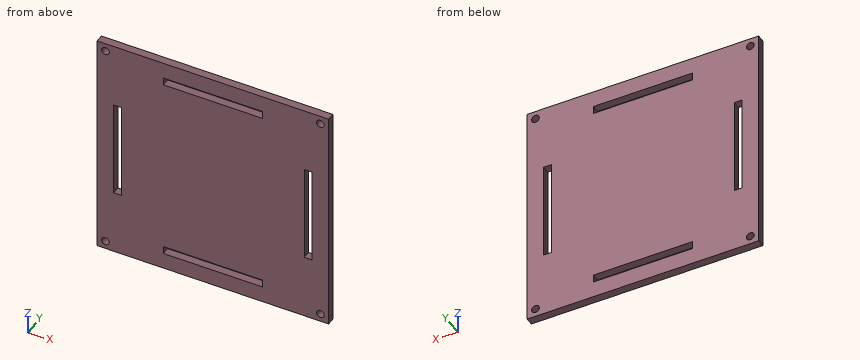
```python
from build123d import *

# Parameters (mm, degrees)
SKETCH_2_W          = 88.9
SKETCH_2_H          = 3
EXTRUDE_1_DEPTH     = 88.9
SKETCH_4_R          = 1.5
CUT_EXTRUDE_1_DEPTH = 3
SKETCH_10_W         = 3
SKETCH_10_H         = 38.1
SKETCH_10_W_2       = 38.1
SKETCH_10_H_2       = 3
CUT_EXTRUDE_6_DEPTH = 3


with BuildPart() as part:
    # 스케치2 → 보스-돌출1 (new body)
    with BuildSketch(Plane.XY):
        Rectangle(SKETCH_2_W, SKETCH_2_H)
    extrude(amount=EXTRUDE_1_DEPTH)

    # 스케치4 → 컷-돌출1 (cut)
    with BuildSketch(Plane(origin=(0, 1.5, 0), x_dir=(1, 0, 0), z_dir=(0, 1, 0))):
        with Locations(Location((-41.275, -85.725, 0), (0, 0, 270))):
            Circle(SKETCH_4_R)
        with Locations(Location((-41.275, -3.175, 0), (0, 0, 270))):
            Circle(SKETCH_4_R)
        with Locations(Location((41.275, -3.175, 0), (0, 0, 270))):
            Circle(SKETCH_4_R)
        with Locations(Location((41.275, -85.725, 0), (0, 0, 270))):
            Circle(SKETCH_4_R)
    extrude(amount=-CUT_EXTRUDE_1_DEPTH, mode=Mode.SUBTRACT)

    # 스케치10 → 컷-돌출6 (cut)
    with BuildSketch(Plane(origin=(0, 1.5, 0), x_dir=(1, 0, 0), z_dir=(0, 1, 0))):
        with Locations((-36.6, -44.45)):
            Rectangle(SKETCH_10_W, SKETCH_10_H)
        with Locations((0, -7.85)):
            Rectangle(SKETCH_10_W_2, SKETCH_10_H_2)
        with Locations((36.6, -44.45)):
            Rectangle(SKETCH_10_W, SKETCH_10_H)
        with Locations((0, -81.05)):
            Rectangle(SKETCH_10_W_2, SKETCH_10_H_2)
    extrude(amount=-CUT_EXTRUDE_6_DEPTH, mode=Mode.SUBTRACT)


solid = part.part
```
Model file for the job. Use its own axes, mm. Round coordinates to 2 decimals unless told otherwise and drop trailing zeros. Order: outer loops, then holes, each group sorted by start corner. A loop starts at its lowest first (then second) coordinate and runs counter-clockwise, first axis right, second up. Notation, with made-up numbers: M 77,73 L 122,73 A24 ccw 122,108 Z; hole C 1,59.5 d4. An arc over 180 degrees is marked long. Use CSV: the item, a comma, the result in double quotes.
Item 1: Saw through at C-C (y = -0.55). State how many separate pieces and enclosed holes the cut face has, plus the area to 3 significant figures.
Worked answers:
separate pieces,"1"
enclosed holes,"8"
area,"7,420 mm²"
Item 2: Probe probe 1 along Z at (x, y) = (5, -0.1); probe 2 along X at (y, z) = (-0.1, 58.5); probe 3 along Z at (x, y) = (36.5, 0.4). List the from-to ranges inside material, lowest first.
Worked answers:
probe 1,"0 to 6.35, 9.35 to 79.55, 82.55 to 88.9"
probe 2,"-44.45 to -38.1, -35.1 to 35.1, 38.1 to 44.45"
probe 3,"0 to 25.4, 63.5 to 88.9"
Item 3: Saw through at B-B (x = 17.5). List the corners of the cut face in (y, z), plus the area to 3 significant figures.
Worked answers:
outline,"M -1.5,0 L 1.5,0 L 1.5,6.35 L -1.5,6.35 Z; M -1.5,9.35 L 1.5,9.35 L 1.5,79.55 L -1.5,79.55 Z; M -1.5,82.55 L 1.5,82.55 L 1.5,88.9 L -1.5,88.9 Z"
area,"249 mm²"
Item 4: Saw through at A-A (z = 53). List the corners of the cut face in (x, y).
Worked answers:
outline,"M -44.45,-1.5 L -38.1,-1.5 L -38.1,1.5 L -44.45,1.5 Z; M -35.1,-1.5 L 35.1,-1.5 L 35.1,1.5 L -35.1,1.5 Z; M 38.1,-1.5 L 44.45,-1.5 L 44.45,1.5 L 38.1,1.5 Z"
